Autodesk Inventor part; units mm, degrees
ref_plane "Work Plane2" through (0, -32.5, -80) normal (0, 0, -1) x (0, 1, 0)
ref_plane "Work Plane1" through (0, 0, 27.5) normal (0, 0, 1) x (1, 0, 0)
ref_plane "Work Plane3" through (0, 0, -200) normal (0, 0, -1) x (-1, 0, 0)
sketch "Sketch11" plane through (0, 0, 0) normal (1, 0, 0) x (0, 1, 0)
  line L0 (-521.0786, 0) -> (2804.4717, 0) construction
  line L1 (0, -249.2) -> (0, 95.2)
  circle A0 centre (0, 0) radius 32.5
  circle A1 centre (0, 0) radius 46
  line L2 (-30, -34.8712) -> (-30, -131.9615)
  line L3 (-30, -131.9615) -> (30, -131.9615)
  line L4 (30, -131.9615) -> (30, -34.8712)
  arc A2 (-30, -131.9615) -> (30, -131.9615) centre (0, -80) ccw
  arc A3 (30, -131.9615) -> (50, -113.1662) centre (0, -80) ccw
  line L5 (0, -160) -> (50, -160)
  line L6 (50, -160) -> (50, -113.1662)
  arc A4 (30, -34.8712) -> (32, -130.7543) centre (2329.3931, -34.8712) ccw
  point P0 (-30, -131.9615)
  point P1 (0, -140)
  point P2 (0, -131.9615)
  point P3 (0, -185.7103)
  point P4 (0, -140)
  point P5 (0, -46)
  dimension "d77" = 65
  dimension "d78" = 92
  dimension "d79" = 60
  dimension "d85" = 20
  dimension "d86" = 20
  dimension "d87" = 60
  dimension "d89" = 32
  dimension "d90" = 140
extrude "Extrusion11" add sketch "Sketch11" along normal mid plane 60 contours L1 A1 L4 L3 | L4 A4 A3
revolve "Revolution1" add sketch "Sketch11" angle 180 mid plane about axis through (0, 0, -10) along (0, 0, 1) picked at (16.8404, -133.4348) contours L1 L3 A2
revolve "Revolution2" cut sketch "Sketch11" angle 360 about axis through (0, 0, -10) along (0, 0, 1) contours L1 A2 A3 L6 L5
mirror "Mirror1" about plane through (0, 0, 0) normal (0, 1, 0)
sketch "Sketch6" plane through (0, 0, 0) normal (1, 0, 0) x (0, 1, 0)
  circle A0 centre (0, 0) radius 32.5
  line L0 (-32.5, 0) -> (-32.5, -80)
  line L1 (-32.5, -80) -> (32.5, -80)
  line L2 (32.5, -80) -> (32.5, 0)
  line L3 (0, 0) -> (0, -80) construction
  line L4 (-32.5, -60) -> (32.5, -60)
  circle A1 centre (0, 0) radius 48.5
  point P0 (32.5, -36)
  point P1 (23.3184, -32.5)
  point P2 (0, -40)
  point P3 (-32.5, -36)
  dimension "d38" = 65
  dimension "d39" = 80
  dimension "d74" = 97
  dimension "d75" = 20
  dimension "d48" = 10
  dimension "d73" = 55
  dimension "d52" = 120
sketch "Sketch5" plane through (0, 0, -171) normal (0, 0, -1) x (-1, 0, 0)
  circle A0 centre (0, 0) radius 10
  point P0 (0, 0)
  dimension "d35" = 20
properties part number "shank_2"
Can you work these out from the model? Positions are in its coordinate system, mm. Give positions to 0.01 mm unless a question says otherwise; leave off trailing zeros. Write each loop counter-clockwise with the first axis right and the second up, starting at its lowest first coordinate (ties: lowest second). Pieces come first, ordered by that corner, then holes. Notation, with made-up numbers: (12.25, 48) -> (23.25, 48) arc R23 cw to (23.25, 62) -> close; hole circle Ø9 at (-3.75, -12). An arc over 180 degrees is marked (long way). One line per item, written item: value.
Q1. Imagine slicing it at B-B on z = -84.5. Please give me the cut outline in (x, y).
Results found:
outline: (-30, -30.54) -> (30, -30.54) -> (30, 30.54) -> (-30, 30.54) -> close
Q2. We'd pull the mould along Y, two halves only. Please class faces 1 (the face through (0, 0, -46)), 2 (the face through (-0.42, -30.486, -82.152)), 3 (the face through (30, 0, -83)), 4 (the face through (-0.42, 30.514, -83.494)): +Y half, -Y half, draft (parallel to the pull), parting line (faces both ways), or undercut.
Results found:
face 1: undercut
face 2: -Y half
face 3: draft
face 4: +Y half
Q3. Please list where these lines run through material, in increasing order: line 1 (Y direction, x = 13, z = -42.5); line 2 (Z direction, x = -10.5, y = 23.5); line 3 (Y direction, x = -2.5, z = -51). Write a range as [from, to].
Results found:
line 1: y = [-30.01, -17.6], [17.6, 30.01]
line 2: z = [-134.2, -39.54]
line 3: y = [-30.06, 30.06]
Q4. Imagine slicing it at A-A on z = -55. Please give me the cut outline in (x, y), and give its area (3 significant figures).
Results found:
outline: (-30, -30.09) -> (30, -30.09) -> (30, 30.09) -> (-30, 30.09) -> close
area: 3,610 mm^2
Q5. For P1, Ø6, axis at x = -18, z = -73.5, coming from the -Y side; P2, Ø10, axis at x = -4, z = -68, coming from the -Y side; P3, Ø6, axis at x = -2, y = 0.5, coming from the +Z side, each with a flat end and sliding along its axis, tell me the tip position at first contact or that it passes through.
Results found:
P1: stops at y = -30.38
P2: stops at y = -30.32
P3: stops at z = -45.87
